Part model, mm, in its own coordinate system. A direction names the side the tool comes from. Round coordinates to 2 decimals unless told otherwise and drop trailing zeros. Order: outer loops, then holes, each group sorted by start corner. A loop starts at its lowest first (then second) coordinate and runs counter-clockwise, first axis right, second up. Notation, with made-up numbers: (31, 74.25) -> (43, 74.25) arc R20 cw to (43, 98.25) -> close; hole circle Ø1 at (35, 55). An arc over 180 degrees is marked (long way). Answer as a JSON object with one key per item and string values. Group by question number.
Autodesk Inventor part; units mm, degrees
ref_plane "YZ Plane" through (0, 0, 0) normal (1, 0, 0) x (0, 1, 0)
ref_plane "XZ Plane" through (0, 0, 0) normal (0, 1, 0) x (-1, 0, 0)
ref_plane "XY Plane" through (0, 0, 0) normal (0, 0, 1) x (1, 0, 0)
sketch "Sketch1" plane through (0, 0, 0) normal (0, 1, 0) x (-1, 0, 0)
  line L0 (0, 0) -> (53.5, 0)
  line L1 (53.5, 0) -> (53.5, 44)
  line L2 (53.5, 44) -> (-19.5, 44)
  line L3 (-19.5, 44) -> (-19.5, 21)
  line L4 (-19.5, 21) -> (0, 0)
  dimension "d3" = 53.5
  dimension "d4" = 44
  dimension "d5" = 23
  dimension "d6" = 73
extrude "Extrusion1" add sketch "Sketch1" along normal mid plane 55
draft "FaceDraft1" angle 20 pull direction (0, 0, -1) faces at (-11.3333, 27.5, 29.3333) (-11.3333, -27.5, 29.3333) fixed edges at (-26.75, 27.5, 0) (-26.75, -27.5, 0)
sketch "Sketch2" plane through (-53.5, 43.5147, 44) normal (0, 0, 1) x (1, 0, 0)
  circle A0 centre (44.2818, -14.0647) radius 1.5
  circle A1 centre (10.2818, -14.0647) radius 1.5
  circle A2 centre (10.2818, -72.9647) radius 1.5
  circle A3 centre (44.2818, -72.9647) radius 1.5
  point P0 (53.5, -43.5147)
extrude "Extrusion2" cut sketch "Sketch2" against normal blind 10.11
sketch "Sketch3" plane through (-53.5, 43.5147, 44) normal (0, 0, 1) x (1, 0, 0)
  circle A0 centre (44.2818, -14.0647) radius 1.5
  circle A1 centre (44.2818, -14.0647) radius 3.25
  circle A2 centre (10.2818, -14.0647) radius 1.5
  circle A3 centre (10.2818, -14.0647) radius 3.25
  circle A4 centre (10.2818, -72.9647) radius 1.5
  circle A5 centre (10.2818, -72.9647) radius 3.25
  circle A6 centre (44.2818, -72.9647) radius 1.5
  circle A7 centre (44.2818, -72.9647) radius 3.25
  point P0 (53.5, -43.5147)
  dimension "d10" = 6.5
extrude "Extrusion3" cut sketch "Sketch3" against normal blind 9
shell "Shell1" thickness 1.5 removed faces 5 at (19.5, -11.7145, 36.3333) at (13, 9.1667, 14) at (-35.6667, 32.8382, 14.6667) at (-35.6667, -32.8382, 14.6667) at (-17.8333, -9.1667, 0)
chamfer "Chamfer1" distance 3 angle 45 4 edges at (-13.9682, -29.45, 42.5) (-47.9682, -29.45, 42.5) (-13.9682, 29.45, 42.5) (-47.9682, 29.45, 42.5)
chamfer "Chamfer2" distance 1 angle 45 4 edges at (-12.2182, -29.45, 33.5) (-46.2182, -29.45, 33.5) (-12.2182, 29.45, 33.5) (-46.2182, 29.45, 33.5)
sketch "Sketch4" plane through (-9.2182, -29.45, 33.89) normal (0, 0, 1) x (1, 0, 0)
  circle A0 centre (0, 0) radius 1.5 construction
  circle A1 centre (-34, 0) radius 1.5 construction
  circle A2 centre (0, 58.9) radius 1.5 construction
  circle A3 centre (-34, 58.9) radius 1.5 construction
  circle A4 centre (-34, 58.9) radius 1.75
  circle A5 centre (0, 58.9) radius 1.75
  circle A6 centre (0, 0) radius 1.75
  circle A7 centre (-34, 0) radius 1.75
  point P0 (9.2182, 29.45)
  dimension "d19" = 3.5
extrude "Extrusion4" cut sketch "Sketch4" along normal through all both and the other way through all
chamfer "Chamfer3" distance 3 angle 45 1 edges at (-52, 0, 42.5)
sketch "Sketch5" plane through (-53.5, -43.5147, 44) normal (-1, 0, 0) x (0, 0, 1)
  line L0 (-33.6389, 49.1201) -> (-11.6389, 49.1201)
  line L1 (-11.6389, 49.1201) -> (-11.6389, 46.3701)
  line L2 (-11.6389, 46.3701) -> (-33.6389, 46.3701)
  line L3 (-33.6389, 46.3701) -> (-33.6389, 49.1201)
  point P0 (-44, 43.5147)
  dimension "d25" = 22
  dimension "d26" = 2.75
extrude "Extrusion5" cut sketch "Sketch5" against normal blind 9
properties part number "Case 2"
Q1. Band-saw the part on D-D (y = -29.45). Count the separate pieces of the cut face and the enclosed holes in it, plus the area to 3 significant figures.
Q2. Two-plate mould, pull along Y, no slides. Class faces 4 (the cylindrical face through (-10.248, -34.087, 36.542)), 5 (the flat face through (-52, -1, 19)), 6 (the cylindrical face through (-41.47, 32.19, 39.56)), 7 (the flat face through (-19.533, 43.255, 43.288)): +Y half, -Y half, draft (parallel to the pull), parting line (faces both ways), or undercut.
Q3. Wall check: line 1 (X direction, y = 26, z = 35); line 2 (X direction, y = -33, z = 37); line 3 (Z direction, x = -34.5, y = -16). Give the ranges that are in metal, low to high. Write a range as [from, to].
Q4. Band-saw the part on A-A (z = 18). List the corners of the cut face in (x, y).
Q5. Band-saw the part on C-C (z = 28.5). List the corners of the cut face in (x, y).
Q6. Drop flat-ended pins along their axis: pin 1 Ø12 at (x, z) = (-11, 32.5) entering from +Y; pin 2 Ø1 at (x, y) = (-19, -11) entering from -Z; pin 3 Ø3 at (x, y) = (-43.5, 31) entering from -Z; pin 4 Ø3 at (x, y) = (-43.22, 29.45) entering from +Z. Give the stop position or say it passes through.
Q7. Which spindle directions (+Z, -Z, +X, -X, +Y, -Y) get a long thin tool onto all of the face, cutting with end or side? Do faces 1 (the flat face through (-46, -33, 33.5)), 2 (the flat face through (-8, -31, 32.39)), 3 (the cylindrical face through (-9.446, 31.185, 33.713)). Say none if no direction does.
Q8. Band-saw the part on B-B (x = -23). List the corners of the cut face in (y, z).
Completed:
{
 "1": {"separate pieces": "3", "enclosed holes": "0", "area": "238 mm2"},
 "2": {"face 4": "undercut", "face 5": "draft", "face 6": "undercut", "face 7": "+Y half"},
 "3": {"line 1": "[-53.5, -52], [-46.48, -39.95], [-12.48, -5.95]", "line 2": "[-53.5, -52], [-46.37, -40.06], [-12.37, -6.06]", "line 3": "[42.5, 44]"},
 "4": {"outline": "(-53.5, -34.05) -> (-52, -34.05) -> (-52, 2.86) -> (-53.5, 2.86) -> close; (-53.5, 5.61) -> (-52, 5.61) -> (-52, 34.05) -> (-53.5, 34.05) -> close"},
 "5": {"outline": "(-53.5, -37.87) -> (-52, -37.87) -> (-52, 2.86) -> (-53.5, 2.86) -> close; (-53.5, 5.61) -> (-52, 5.61) -> (-52, 37.87) -> (-53.5, 37.87) -> close"},
 "6": {"pin 1": "y = 34.2", "pin 2": "z = 42.5", "pin 3": "z = 32.39", "pin 4": "through"},
 "7": {"face 1": "-Z", "face 2": "-Z, +X, +Y, -Y", "face 3": "+Z, -Z"},
 "8": {"outline": "(-43.51, 44) -> (-42.97, 42.5) -> (42.97, 42.5) -> (43.51, 44) -> close"}
}
